from build123d import *

# Parameters (mm, degrees)
BOSS_EXTRUDE1_DEPTH      = 8.509
BOSS_EXTRUDE1_DEPTH_BACK = 8.509
SKETCH3_R                = 15.519490552
BOSS_EXTRUDE2_DEPTH      = 38.1
SKETCH4_R                = 10.825000036
CUT_EXTRUDE1_DEPTH       = 31.75
CUT_EXTRUDE2_DEPTH       = 73.611468784
CUT_EXTRUDE2_DEPTH_BACK  = 73.611468784
SKETCH5_W                = 9.906
SKETCH5_H                = 56.435801088
SKETCH6_R                = 5.08
CUT_EXTRUDE3_DEPTH       = 75.892851262
CHAMFER1_SIZE            = 0.254
CHAMFER2_SIZE            = 0.508
FILLET1_R                = 1.27
FILLET2_R                = 1.27
SKETCH11_R               = 15.519490552
CUT_EXTRUDE4_DEPTH       = 45.520887291
FILLET4_R                = 2.54
SKETCH12_R               = 2.3495
CUT_EXTRUDE5_DEPTH       = 44.969525515
CUT_EXTRUDE6_START       = 31.75
SKETCH13_R               = 10.875012636
CUT_EXTRUDE6_DEPTH       = 23.876
CUT_EXTRUDE7_START       = 23.876
SKETCH14_R               = 10.925012636
CUT_EXTRUDE7_DEPTH       = 16.002


with BuildPart() as part:
    # Sketch2 → Boss-Extrude1 (new, two sides: drawn at the far end of the back side and taken through both)
    with BuildSketch(Plane.XY.offset(-BOSS_EXTRUDE1_DEPTH_BACK)):
        with BuildLine():
            Line((11.43, -31.115), (7.565118148, 0.912900544))
            ThreePointArc((7.565118148, 0.912900544), (0, 7.62), (-7.565118148, 0.912900544))
            Line((-7.565118148, 0.912900544), (-11.43, -31.115))
            Line((-11.43, -31.115), (11.43, -31.115))
        make_face()
    extrude(amount=BOSS_EXTRUDE1_DEPTH + BOSS_EXTRUDE1_DEPTH_BACK)

    # Sketch3 → Boss-Extrude2 (add)
    with BuildSketch(Plane.XZ.offset(31.115)):
        with Locations(Location((0, 0, 0), (0, 0, 180))):
            Circle(SKETCH3_R)
    extrude(amount=BOSS_EXTRUDE2_DEPTH)

    # Sketch4 → Cut-Extrude1 (cut)
    with BuildSketch(Plane.XZ.offset(69.215)):
        Circle(SKETCH4_R)
    extrude(amount=-CUT_EXTRUDE1_DEPTH, mode=Mode.SUBTRACT)

    # Sketch5 → Cut-Extrude2 (cut, two sides: drawn at the far end of the back side and taken through both)
    with BuildSketch(Plane(origin=(0, 0, 0), x_dir=(0, 0, -1), z_dir=(1, 0, 0)).offset(-CUT_EXTRUDE2_DEPTH_BACK)):
        with Locations((0, 0.912900544)):
            Rectangle(SKETCH5_W, SKETCH5_H)
    extrude(amount=CUT_EXTRUDE2_DEPTH + CUT_EXTRUDE2_DEPTH_BACK, mode=Mode.SUBTRACT)

    # Sketch6 → Cut-Extrude3 (cut, through all)
    with BuildSketch(Plane(origin=(0, 0, -8.509), x_dir=(-1, 0, 0), z_dir=(0, 0, -1))):
        with Locations(Location((0, 0, 0), (0, 0, 180))):
            Circle(SKETCH6_R)
    extrude(amount=-CUT_EXTRUDE3_DEPTH, mode=Mode.SUBTRACT)

    # Chamfer1
    chamfer1_edges = [part.edges().sort_by_distance(p)[0] for p in [
        (-5.08, 0, 8.509),
        (-5.08, 0, -4.953),
        (-5.08, 0, 4.953),
        (-5.08, 0, -8.509),
    ]]
    chamfer(chamfer1_edges, length=CHAMFER1_SIZE)

    # Chamfer2
    chamfer2_edges = [part.edges().sort_by_distance(p)[0] for p in [
        (-10.825000036, -69.215, 0),
    ]]
    chamfer(chamfer2_edges, length=CHAMFER2_SIZE)

    # Fillet1
    fillet1_edges = [part.edges().sort_by_distance(p)[0] for p in [
        (-9.497559074, -15.101049728, -8.509),
        (9.497559074, -15.101049728, -8.509),
        (0, 7.62, -8.509),
        (-9.497559074, -15.101049728, 8.509),
        (9.497559074, -15.101049728, 8.509),
        (0, 7.62, 8.509),
    ]]
    fillet(fillet1_edges, radius=FILLET1_R)

    # Fillet2
    fillet2_edges = [part.edges().sort_by_distance(p)[0] for p in [
        (11.43, -31.115, 0),
        (-11.43, -31.115, 0),
        (11.053691049, -31.115, -8.138646936),
        (11.053691049, -31.115, 8.138646936),
        (-11.053691049, -31.115, -8.138646936),
        (-11.053691049, -31.115, 8.138646936),
        (0, -31.115, -8.509),
        (0, -31.115, 8.509),
    ]]
    fillet(fillet2_edges, radius=FILLET2_R)

    # Sketch11 → Cut-Extrude4 (cut, through all)
    with BuildSketch(Plane(origin=(0, -31.115, 0), x_dir=(1, 0, 0), z_dir=(0, 1, 0))):
        with Locations(Location((0, 0, 0), (0, 0, 180))):
            Circle(SKETCH11_R)
    extrude(amount=CUT_EXTRUDE4_DEPTH, mode=Mode.SUBTRACT)

    # Fillet4
    fillet4_edges = [part.edges().sort_by_distance(p)[0] for p in [
        (15.519490552, -31.115, 0),
    ]]
    fillet(fillet4_edges, radius=FILLET4_R)

    # Sketch12 → Cut-Extrude5 (cut, through all)
    with BuildSketch(Plane(origin=(0, -31.115, 0), x_dir=(1, 0, 0), z_dir=(0, 1, 0))):
        with Locations(Location((0, 0, 0), (0, 0, 180))):
            Circle(SKETCH12_R)
    extrude(amount=-CUT_EXTRUDE5_DEPTH, mode=Mode.SUBTRACT)

    # Sketch13 → Cut-Extrude6 (cut)
    with BuildSketch(Plane.XZ.offset(37.465).offset(CUT_EXTRUDE6_START)):
        Circle(SKETCH13_R)
    extrude(amount=-CUT_EXTRUDE6_DEPTH, mode=Mode.SUBTRACT)

    # Sketch14 → Cut-Extrude7 (cut)
    with BuildSketch(Plane.XZ.offset(45.339).offset(CUT_EXTRUDE7_START)):
        Circle(SKETCH14_R)
    extrude(amount=-CUT_EXTRUDE7_DEPTH, mode=Mode.SUBTRACT)


solid = part.part
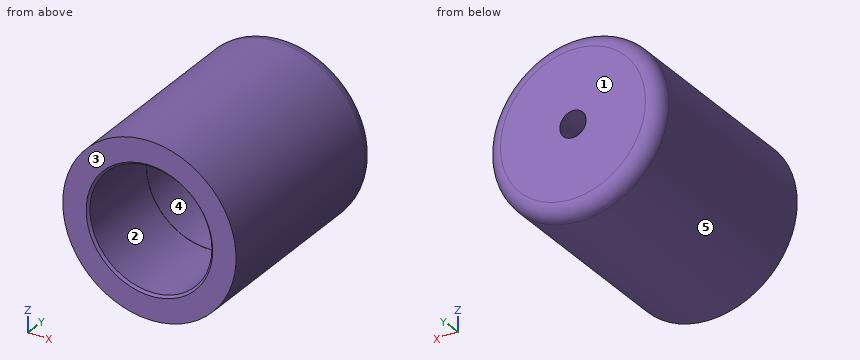
Geometry: final body of the model. Coordinates: model frame, mm. Face numbers are marked on the shaded views. A direction names the side the tool comes from. Coordinates: 2 decimals unless noted, no trailing zeros. Order: outer loops, then holes, each group sorted by start corner. A loop starts at its lowest first (then second) coordinate and runs counter-clockwise, first axis right, second up. Notation, with made-up numbers: (79.25, 21) - (87.25, 21) arc R11 cw to (87.25, 34) - close; hole circle Ø6 at (-17, 33.5). An arc over 180 degrees is marked (long way). Use one line per item in the form item = value.
1) Set-up query: the marked faces 1 and 2. Return all of +Z, -Z, +X, -X, +Y, -Y with unobstructed straight access to the full face (end or side cutting, diameter ignored); none if empty.
Solutions:
face_1 = +Z, -Z, +X, -X, +Y
face_2 = -Y
2) Pin query (flat end, axial travel): pin 1 (11 mm diameter, centred on x = 1, z = 3.5, fed in from -Y) (3 decimals); pin 2 (12 mm diameter, centred on y = -50, z = 10, fed in from -X); pin 3 (4 mm diameter, centred on x = -11, y = -38.5, fed in from -Z); pin 4 (4 mm diameter, centred on x = 0, z = 0, fed in from +Y). Return the tip coordinate at first contact, or that it passes through.
Solutions:
pin_1 = -37.465
pin_2 = -15
pin_3 = -12.64
pin_4 = through
3) Ray query, L1, parallel to Z at x = 0, y = -50.25; L2, parallel to Z at x = 0, y = -42 (1 decimal); L3, parallel to Y at x = -0.5, z = -8.5 (3 decimals). Return the intervals inside material, ascending.
Solutions:
L1 = -15.52 to -10.88, 10.88 to 15.52
L2 = -15.5 to -10.8, 10.8 to 15.5
L3 = -37.465 to -31.115
4) Section D-D (y = -61). Return loops of the section in (x, z).
Solutions:
outline = circle Ø31.04 at (0, 0); hole circle Ø21.85 at (0, 0)
5) Mould query, pull axis X, two halves, no side actions, for the marked faces 3, 4 and 5. Classes: +X half, -X half, draft (parallel to the pull), parting line (faces both ways), or undercut.
Solutions:
face_3 = draft
face_4 = undercut
face_5 = parting line
